Can you work these out from the drawing? Everything is in mm from the part's minimum corner. A direction names the side the tool comes from. Give positions to 0.01 mm unless a question says otherwise; leave off trailing zeros. Write each loop counter-clockwise with the first axis right and the second up, starting at its lowest first coordinate (ties: lowest second). Pieces come first, ordered by that corner, then holes. Notation, with made-up numbers: (-24, -36) - (13, -36) arc R28 ccw to (13, -4) - close; hole circle Ø5 at (-9, 63). An arc over 180 degrees is marked (long way). Return JSON: item names as keys, results as strings. Group by question number.
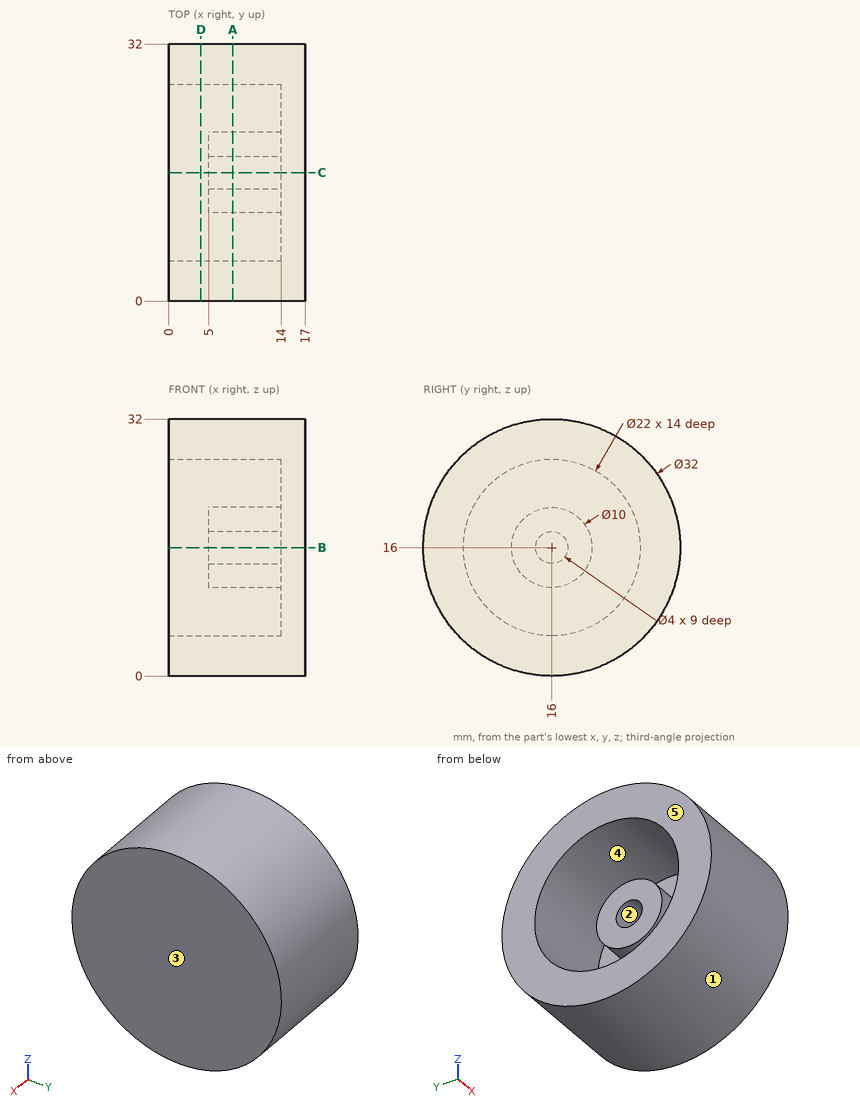
1) I need wall thicknesses on line 1 along Y through (x, z) = (11.5, 16); line 2 along Y through (x, z) = (9.75, 12). Which ranges of each line are inside material? Lowest first, please.
2) We'd pull the mould along Z, two halves only. Please class the marked faces 1, 2 and 3: pulls with the +Z half, pulls with the -Z half, needs draft (parallel to the pull), parting line crosses it, or undercut.
3) Imagine slicing it at A-A, the plane x = 8. Write out the boundary of the cut face in (y, z).
4) On a 3-axis mill with a long thin cutter (end or side, diameter ignored), from which of +Z, -Z, +X, -X, +Y, -Y can I reach the whole of each face in a straight line? I mean the marked faces 4 and 5. Say none if no direction works.
5) Will these pins go through, and if not, where does the flat tip stop? pin 1 Ø6 at (y, z) = (17.5, 17) entering from -X; pin 2 Ø1.5 at (y, z) = (7, 17.5) entering from -X; pin 3 Ø5 at (x, z) = (10.5, 6) entering from -Y.
6) Imagine slicing it at B-B, the plane z = 16. Write out the boundary of the cut face in (x, y).
7) Imagine slicing it at D-D, the plane x = 4. Write out the boundary of the cut face in (y, z), and give its area (3 significant figures).
Resolved:
{
 "1": {"line 1": "0 to 5, 11 to 14, 18 to 21, 27 to 32", "line 2": "0.51 to 5.75, 13 to 19, 26.25 to 31.49"},
 "2": {"face 1": "parting line crosses it", "face 2": "undercut", "face 3": "needs draft"},
 "3": {"outline": "circle Ø32 at (16, 16); circle Ø10 at (16, 16); hole circle Ø22 at (16, 16); hole circle Ø4 at (16, 16)"},
 "4": {"face 4": "-X", "face 5": "+Z, -Z, -X, +Y, -Y"},
 "5": {"pin 1": "x = 5", "pin 2": "x = 14", "pin 3": "y = 1.87"},
 "6": {"outline": "(0, 0) - (17, 0) - (17, 32) - (0, 32) - (0, 27) - (14, 27) - (14, 21) - (5, 21) - (5, 18) - (14, 18) - (14, 14) - (5, 14) - (5, 11) - (14, 11) - (14, 5) - (0, 5) - close"},
 "7": {"outline": "circle Ø32 at (16, 16); hole circle Ø22 at (16, 16)", "area": "424 mm^2"}
}
